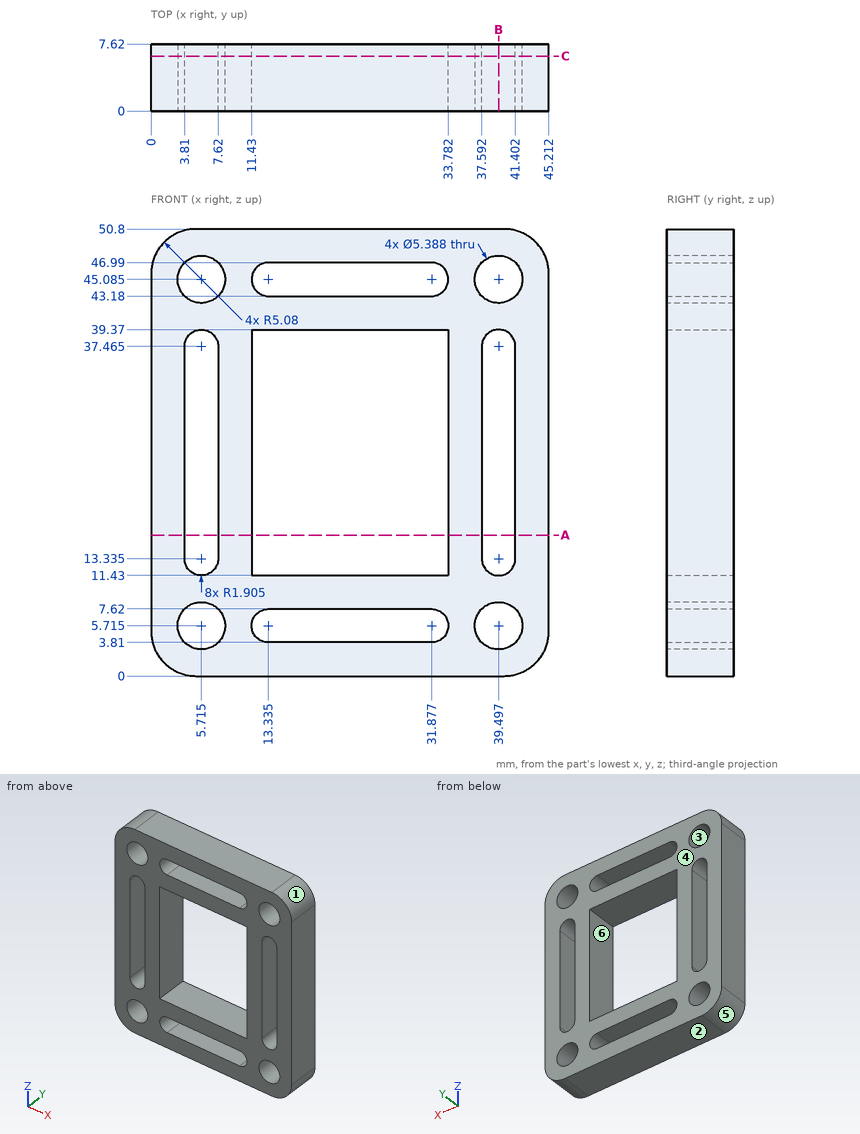
Verification items for this drawing (mm, ordinates from the low corner). A direction names the side the tool comes from. Give positions to 0.01 mm unless a question says otherwise; leave off trailing zeros. Write each loop counter-clockwise with the first axis right and the second up, starting at its lowest first coordinate (ties: lowest second). Pieces come first, ordered by that corner, then holes. Notation, with made-up numbers: (-20, 50) -> (20, 50) arc R28 cw to (20, 83) -> close; hole circle Ø6 at (-40, 31.5). An arc over 180 degrees is marked (long way). Use one line per item in the form item = value.
Item 1: Mould release check, pull along Z, two halves, no side actions. Record for the marked faces 1, 2, 3 and 4: released by +Z, released by -Z, zero draft, split by the parting line, or undercut.
Results list:
face_1 = released by +Z
face_2 = released by -Z
face_3 = undercut
face_4 = zero draft
Item 2: Sectioned sample at B-B on x = 39.5. Enter the section's corners in (y, z), plus the area to 3 significant figures.
Results list:
outline = (0, 0) -> (7.62, 0) -> (7.62, 3.02) -> (0, 3.02) -> close; (0, 8.41) -> (7.62, 8.41) -> (7.62, 11.43) -> (0, 11.43) -> close; (0, 39.37) -> (7.62, 39.37) -> (7.62, 42.39) -> (0, 42.39) -> close; (0, 47.78) -> (7.62, 47.78) -> (7.62, 50.8) -> (0, 50.8) -> close
area = 92.1 mm2
Item 3: Sectioned sample at A-A on z = 16. Enter the section's corners in (x, y).
Results list:
outline = (0, 0) -> (3.81, 0) -> (3.81, 7.62) -> (0, 7.62) -> close; (7.62, 0) -> (11.43, 0) -> (11.43, 7.62) -> (7.62, 7.62) -> close; (33.78, 0) -> (37.59, 0) -> (37.59, 7.62) -> (33.78, 7.62) -> close; (41.4, 0) -> (45.21, 0) -> (45.21, 7.62) -> (41.4, 7.62) -> close
Item 4: Access from +Z, -Z, +X, -X, +Y, -Y to the whole of each face (thin tool, end or side, straight path). Record for the marked faces 5 and 6.
Results list:
face_5 = -Z, -X, +Y, -Y
face_6 = +Y, -Y
Item 5: Sectioned sample at C-C on y = 6.25. Count the separate pieces of the cut face and the enclosed holes in it, plus the area to 3 significant figures.
Results list:
separate_pieces = 1
enclosed_holes = 9
area = 1,190 mm2
Item 6: Depth check by flat-ended pin: pin 1 Ø5 at (x, z) = (39.497, 45.085) entering from +Y. Enter the tip coordinate at first touch or a pass-through.
Results list:
pin_1 = through
Item 7: Scan lines: line 1 (X direction, y = 4.25, z = 26.5); line 2 (Z direction, x = 15, y = 5.5); line 3 (Z direction, x = 7, y = 3.5). Record each from-to range of solid material in increasing order.
Results list:
line_1 = 0 to 3.81, 7.62 to 11.43, 33.78 to 37.59, 41.4 to 45.21
line_2 = 0 to 3.81, 7.62 to 11.43, 39.37 to 43.18, 46.99 to 50.8
line_3 = 0 to 3.35, 8.08 to 11.93, 38.87 to 42.72, 47.45 to 50.8
